Geometry: final body of the model. Coordinates: model frame, mm. A direction names the side the tool comes from. Coordinates: 2 decimals unless noted, no trailing zeros. Order: outer loops, then holes, each group sorted by start corner. A loop starts at its lowest first (then second) coordinate and runs counter-clockwise, first axis right, second up. Notation, with made-up numbers: M 0,13.5 L 45,13.5 A19 ccw 45,18.5 Z; hole C 69.25,66 d7. An arc over 180 degrees is marked long. Use CSV: the item, a comma, the result in double quotes. Start each with the question number.
1. Pull-direction query (X, two-part tool) for faces 4 (the cylindrical face through (-34.02, 6.62, -0.94)), 5 (the flat face through (-6.35, -6, 47)), 6 (the cylindrical face through (-30.235, 12.522, 23.183)), 7 (the flat face through (-47, -6, 6.35)); classes: pulls with the +X half, pulls with the -X half, needs draft (parallel to the pull), parting line crosses it, or undercut.
2. Material intervals for line 1 (Y direction, x = 7.5, z = 41); line 2 (X direction, y = 20.5, z = -4); line 3 (X direction, y = 4.5, z = -1), sorted ascending.
3. Section query B-B on x = 0. Return the cut outline in (y, z), and give its area (3 significant figures).
4. Section query D-D on z = 31.75. Return the cut outline in (x, y), and give its area (3 significant figures).
5. Section query C-C on y = -9. Return the cut outline in (x, z), and give its area (3 significant figures).
6. Section query A-A on z = 0. Return the cut outline in (x, y).
7. First-contact query: P1, Ø2, axis at x = -20.5, y = -5.5, coming from the +Z side; P2, Ø5, axis at y = -9.5, z = -48, coming from the +X side; P3, Ø2, axis at y = 19.5, z = 18.5, coming from the -X side. Flat tips, straight axial feed; report the tip coordinate or a pass-through.
8. Set-up query: faces 1 (the flat face through (-47, -6, -6.35)), 2 (the flat face through (6.35, -6, -47)), 3 (the flat face through (47, -6, 6.35)). Return all of +Z, -Z, +X, -X, +Y, -Y with unobstructed straight access to the full face (end or side cutting, diameter ignored); none if empty.
from build123d import *

# Parameters (mm, degrees)
SKETCH2_R                    = 38.1
SKETCH2_R_2                  = 6.35
BOSS_EXTRUDE2_DEPTH          = 25.4
SKETCH2_5_R                  = 6.35
BOSS_EXTRUDE3_DEPTH          = 12.7
F_10_0_1935_DIAMETER_HOLE2_D = 4.9149
CIRPATTERN2_COUNT            = 4


with BuildPart() as part:
    # Sketch2 → Boss-Extrude2 (new body)
    with BuildSketch(Plane(origin=(0, 0, 0), x_dir=(1, 0, 0), z_dir=(0, 1, 0))):
        Circle(SKETCH2_R)
        Circle(SKETCH2_R_2, mode=Mode.SUBTRACT)
    extrude(amount=BOSS_EXTRUDE2_DEPTH)

    # Sketch2_5 → Boss-Extrude3 (add)
    with BuildSketch(Plane(origin=(0, 0, 0), x_dir=(1, 0, 0), z_dir=(0, 1, 0))):
        with BuildLine():
            Line((-6.35, 50.401562476), (-6.35, 43.994090512))
            ThreePointArc((-6.35, 43.994090512), (-31.430896424, 31.430896424), (-43.994090512, 6.35))
            Line((-43.994090512, 6.35), (-50.401562476, 6.35))
            ThreePointArc((-50.401562476, 6.35), (-50.8, 0), (-50.401562476, -6.35))
            Line((-50.401562476, -6.35), (-43.994090512, -6.35))
            ThreePointArc((-43.994090512, -6.35), (-31.430896424, -31.430896424), (-6.35, -43.994090512))
            Line((-6.35, -43.994090512), (-6.35, -50.401562476))
            ThreePointArc((-6.35, -50.401562476), (0, -50.8), (6.35, -50.401562476))
            Line((6.35, -50.401562476), (6.35, -43.994090512))
            ThreePointArc((6.35, -43.994090512), (31.430896424, -31.430896424), (43.994090512, -6.35))
            Line((43.994090512, -6.35), (50.401562476, -6.35))
            ThreePointArc((50.401562476, -6.35), (50.8, 0), (50.401562476, 6.35))
            Line((50.401562476, 6.35), (43.994090512, 6.35))
            ThreePointArc((43.994090512, 6.35), (31.430896424, 31.430896424), (6.35, 43.994090512))
            Line((6.35, 43.994090512), (6.35, 50.401562476))
            ThreePointArc((6.35, 50.401562476), (0, 50.8), (-6.35, 50.401562476))
        make_face()
        Circle(SKETCH2_5_R, mode=Mode.SUBTRACT)
    extrude(amount=-BOSS_EXTRUDE3_DEPTH)

    # 10 _0.1935_ Diameter Hole2 (through all)
    with Locations(Plane(origin=(0, -12.7, 31.75), x_dir=(0, 0, -1), z_dir=(0, -1, 0))):
        with Locations((0, 0)):
            f_10_0_1935_diameter_hole2 = Hole(F_10_0_1935_DIAMETER_HOLE2_D / 2)

    # CirPattern2: 10 _0.1935_ Diameter Hole2 ×4 about axis
    cirpattern2_axis = Axis((0, 0, 0), (0, 1, 0))
    for i in range(1, CIRPATTERN2_COUNT):
        add(f_10_0_1935_diameter_hole2.rotate(cirpattern2_axis, i * 360 / CIRPATTERN2_COUNT), mode=Mode.SUBTRACT)


solid = part.part
Results list:
1,face 4,"undercut"
1,face 5,"pulls with the -X half"
1,face 6,"parting line crosses it"
1,face 7,"needs draft"
2,line 1,"y = -12.7 to 0"
2,line 2,"x = -37.89 to -4.93, 4.93 to 37.89"
2,line 3,"x = -38.09 to -33.99, -29.51 to -6.27, 6.27 to 29.51, 33.99 to 38.09"
3,outline,"M -12.7,-50.8 L 0,-50.8 L 0,-38.1 L 25.4,-38.1 L 25.4,-34.21 L -12.7,-34.21 Z; M -12.7,-29.29 L 25.4,-29.29 L 25.4,-6.35 L -12.7,-6.35 Z; M -12.7,6.35 L 25.4,6.35 L 25.4,29.29 L -12.7,29.29 Z; M -12.7,34.21 L 25.4,34.21 L 25.4,38.1 L 0,38.1 L 0,50.8 L -12.7,50.8 Z"
3,area,"2,370 mm²"
4,outline,"M -31.11,-12.7 L -2.46,-12.7 L -2.46,25.4 L -21.06,25.4 L -21.06,0 L -31.11,0 Z; M 2.46,-12.7 L 31.11,-12.7 L 31.11,0 L 21.06,0 L 21.06,25.4 L 2.46,25.4 Z"
4,area,"1,670 mm²"
5,outline,"M -50.4,-6.35 L -43.99,-6.35 A44.45 ccw -6.35,-43.99 L -6.35,-50.4 A50.8 ccw 6.35,-50.4 L 6.35,-43.99 A44.45 ccw 43.99,-6.35 L 50.4,-6.35 A50.8 ccw 50.4,6.35 L 43.99,6.35 A44.45 ccw 6.35,43.99 L 6.35,50.4 A50.8 ccw -6.35,50.4 L -6.35,43.99 A44.45 ccw -43.99,6.35 L -50.4,6.35 A50.8 ccw Z; hole C -31.75,0 d4.91; hole C 0,0 d12.7; hole C 0,-31.75 d4.91; hole C 0,31.75 d4.91; hole C 31.75,0 d4.91"
5,area,"6,330 mm²"
6,outline,"M -50.8,-12.7 L -34.21,-12.7 L -34.21,25.4 L -38.1,25.4 L -38.1,0 L -50.8,0 Z; M -29.29,-12.7 L -6.35,-12.7 L -6.35,25.4 L -29.29,25.4 Z; M 6.35,-12.7 L 29.29,-12.7 L 29.29,25.4 L 6.35,25.4 Z; M 34.21,-12.7 L 50.8,-12.7 L 50.8,0 L 38.1,0 L 38.1,25.4 L 34.21,25.4 Z"
7,P1,"stops at z = 39.94"
7,P2,"stops at x = 6.35"
7,P3,"stops at x = -33.84"
8,face 1,"-Z, -X, +Y, -Y"
8,face 2,"-Z, +X, +Y, -Y"
8,face 3,"+Z, +X, +Y, -Y"
